```python
from build123d import *

# Parameters (mm, degrees)
SKETCH159_W     = 24
SKETCH159_H     = 5.5
PAD063_DEPTH    = 14
SKETCH160_R     = 4.75
PAD064_DEPTH    = 24
SKETCH161_R     = 3
POCKET063_DEPTH = 24.001
SKETCH162_W     = 20
SKETCH162_H     = 1.5
POCKET064_DEPTH = 12
SKETCH163_R     = 2
POCKET065_DEPTH = 7.501
SKETCH164_W     = 4.75
SKETCH164_H     = 1
PAD065_DEPTH    = 1
SKETCH166_W     = 4.75
SKETCH166_H     = 1
POCKET066_DEPTH = 4.751
FILLET011_R     = 2


with BuildPart() as part:
    # Sketch159 → Pad063 (new body)
    with BuildSketch(Plane.XY):
        with Locations((12, 2.75)):
            Rectangle(SKETCH159_W, SKETCH159_H)
    extrude(amount=PAD063_DEPTH)

    # Sketch160 (on Face6 of Pad063) → Pad064 (join)
    with BuildSketch(Plane.XY.offset(14)):
        with Locations((12, 2.75)):
            Circle(SKETCH160_R)
    extrude(amount=-PAD064_DEPTH)

    # Sketch161 (on Face7 of Pad064) → Pocket063 (cut, through all)
    with BuildSketch(Plane.XY.offset(14)):
        with Locations((12, 2.75)):
            Circle(SKETCH161_R)
    extrude(amount=-POCKET063_DEPTH, mode=Mode.SUBTRACT)

    # Sketch162 (on Face5 of Pocket063) → Pocket064 (cut)
    with BuildSketch(Plane.XY.offset(14)):
        with Locations((12, 2.75)):
            Rectangle(SKETCH162_W, SKETCH162_H)
    extrude(amount=-POCKET064_DEPTH, mode=Mode.SUBTRACT)

    # Sketch163 (on Face2 of Pocket064) → Pocket065 (cut, through all)
    with BuildSketch(Plane(origin=(0, 5.5, 0), x_dir=(-1, 0, 0), z_dir=(0, 1, 0))):
        with Locations((-19.3, 4.7)):
            Circle(SKETCH163_R)
        with Locations((-4.7, 4.7)):
            Circle(SKETCH163_R)
    extrude(amount=-POCKET065_DEPTH, mode=Mode.SUBTRACT)

    # Sketch164 (on Face19 of Pocket065) → Pad065 (join)
    with BuildSketch(Plane(origin=(0, 0, -10), x_dir=(1, 0, 0), z_dir=(0, 0, -1))):
        with Locations((9.625, -2.25)):
            Rectangle(SKETCH164_W, SKETCH164_H)
    extrude(amount=PAD065_DEPTH)

    # Sketch165 (on Face24 of Pad065) → Groove (revolve, cut)
    with BuildSketch(Plane(origin=(0, 2.75, 0), x_dir=(-1, 0, 0), z_dir=(0, 1, 0))):
        Polygon((-7.25, -1.982419), (-8.25, -3.986814), (-7.25, -3.986814), (-8.25, -5.99121), (-7.25, -5.99121), (-8.25, -7.995605), (-7.25, -7.995605), (-8.25, -10), (-7.25, -10), (-6.25, -10), (-6.25, -1.982419), align=None)
    revolve(axis=Axis((11.996907, 2.75, -10.00717), (0, 0, 1)), mode=Mode.SUBTRACT)

    # Sketch166 (on Face37 of Groove) → Pocket066 (cut, through all)
    with BuildSketch(Plane(origin=(0, 2.75, 0), x_dir=(-1, 0, 0), z_dir=(0, 1, 0))):
        with Locations((-9.625, -10.5)):
            Rectangle(SKETCH166_W, SKETCH166_H)
    extrude(amount=-POCKET066_DEPTH, mode=Mode.SUBTRACT)

    # Fillet011
    fillet011_edges = [part.edges().sort_by_distance(p)[0] for p in [
        (0, 5.5, 7),
        (0, 0, 7),
        (24, 5.5, 7),
        (24, 0, 7),
    ]]
    fillet(fillet011_edges, radius=FILLET011_R)


solid = part.part
```
Work out the finished part from the listing and answer in its coordinate system (mm). A direction names the side the tool comes from. Coordinates: 2 decimals unless noted, no trailing zeros. Loops run counter-clockwise (first coordinate to the right, second up) from the corner with the lowest first, then second, coordinate; pieces in that order, holes last. Notation, with made-up numbers: (-34.5, -3) - (-16.5, -3) arc R23 cw to (-16.5, 18) - close; hole circle Ø8 at (-39.5, 5.25). An arc over 180 degrees is marked (long way). Use a Markdown table: item, result.
Item 1: Consider probe 1 along Z at (x, y) = (19.3, 4.95); probe 2 along Y at (x, z) = (2.75, 5.5); probe 3 along Z at (x, y) = (11, -1.25). Determine where each line is inside the solid, lowest interval first. Write a range as from..to.
Evaluation:
| item | result |
|---|---|
| probe 1 | z = 0..2.7, 6.7..14 |
| probe 2 | y = 0..2, 3.5..5.5 |
| probe 3 | z = -9.25..-8, -7.24..-5.99, -5.24..-3.99, -3.23..14 |
Item 2: For faces 4 (the flat face through (5, 2, 8)), 5 (the flat face through (8, 4, -7.996)), 6 (the flat face through (5, 5.5, 7)), determine the directions among +Z, -Z, +X, -X, +Y, -Y from which every point of the face is accessible in a straight line to the end or side of a thin tool.
Evaluation:
| item | result |
|---|---|
| face 4 | +Z |
| face 5 | none |
| face 6 | +Z, -Z, -X, +Y |
Item 3: The mould has two halves that part along Y. Classify faces 1 (the cylindrical face through (0.57, 4.9, 7.1)), 2 (the flat face through (5, 3, 2)), 3 (the cylindrical face through (2.792, 1.014, 5.301)): +Y half, -Y half, draft (parallel to the pull), parting line (faces both ways), or undercut.
Evaluation:
| item | result |
|---|---|
| face 1 | +Y half |
| face 2 | undercut |
| face 3 | draft |
Item 4: Find section C-C, the plane z = 1.5. Determine the outline of the cut face in (x, y), and give its area (3 significant figures).
Evaluation:
| item | result |
|---|---|
| outline | (0, 2) arc R2 ccw to (2, 0) - (8.13, 0) arc R4.75 ccw to (15.87, 0) - (22, 0) arc R2 ccw to (24, 2) - (24, 3.5) arc R2 ccw to (22, 5.5) - (15.87, 5.5) arc R4.75 ccw to (8.13, 5.5) - (2, 5.5) arc R2 ccw to (0, 3.5) - close; hole circle Ø6 at (12, 2.75) |
| area | 122 mm2 |
Item 5: Find section B-B, the plane z = 7. Determine the outline of the cut face in (x, y).
Evaluation:
| item | result |
|---|---|
| outline | (0, 2) arc R2 ccw to (2, 0) - (8.13, 0) arc R4.75 ccw to (15.87, 0) - (22, 0) arc R2 ccw to (24, 2) - (24, 3.5) arc R2 ccw to (22, 5.5) - (15.87, 5.5) arc R4.75 ccw to (8.13, 5.5) - (2, 5.5) arc R2 ccw to (0, 3.5) - close; hole (2, 2) - (9.1, 2) arc R3 ccw to (14.9, 2) - (22, 2) - (22, 3.5) - (14.9, 3.5) arc R3 ccw to (9.1, 3.5) - (2, 3.5) - close |
Item 6: Given pin 1 Ø1.6 at (x, y) = (3.5, 3.5) entering from -Z; pin 2 Ø2 at (x, z) = (20, 9.5) entering from +Y; pin 3 Ø5.5 at (x, z) = (7, 8.5) entering from +Y, each flat-ended and moving along its own axis, determine where each tip first touches the part or whether it passes through.
Evaluation:
| item | result |
|---|---|
| pin 1 | stops at z = 0 |
| pin 2 | stops at y = 5.5 |
| pin 3 | stops at y = 6.93 |
Item 7: Find section A-A, the plane x = 4.7. Determine the outline of the cut face in (y, z), and give its area (3 significant figures).
Evaluation:
| item | result |
|---|---|
| outline | (0, 0) - (5.5, 0) - (5.5, 2.7) - (3.5, 2.7) - (3.5, 2) - (2, 2) - (2, 2.7) - (0, 2.7) - close; (0, 6.7) - (2, 6.7) - (2, 14) - (0, 14) - close; (3.5, 6.7) - (5.5, 6.7) - (5.5, 14) - (3.5, 14) - close |
| area | 43.0 mm2 |
Item 8: Find section D-D, the plane x = 17.75. Determine the outline of the cut face in (y, z).
Evaluation:
| item | result |
|---|---|
| outline | (0, 0) - (5.5, 0) - (5.5, 3.44) - (3.5, 3.44) - (3.5, 2) - (2, 2) - (2, 3.44) - (0, 3.44) - close; (0, 5.96) - (2, 5.96) - (2, 14) - (0, 14) - close; (3.5, 5.96) - (5.5, 5.96) - (5.5, 14) - (3.5, 14) - close |
